Geometry: see drawing. Coordinates: mm, zero at the bounding-box minimum. Give positions to 0.01 mm unless a question says otherwise; leave off trailing zeros. Write each loop counter-clockwise with the first axis right and the second up, starting at its lowest first coordinate (ties: lowest second). Pieces come first, ordered by that corner, then holes. Notation, with made-up numbers: (66, 75) - (87, 75) arc R21 cw to (87, 113) - close; hole circle Ø9 at (7, 32). An arc over 180 degrees is marked (long way). Use a Markdown table: item, result. Add a question column.
1. Section query A-A, the plane y = 20.5. Return loops of the section in (x, z).
2. Section query B-B, the plane x = 85. Return loops of the section in (y, z).
3. Section query D-D, the plane y = 9.5. Return loops of the section in (x, z).
4. Pin query (flat end, axial travel): pin 1 (2 mm diameter, centred on x = 94.53, y = 4, fed in from -Z); pin 2 (3 mm diameter, centred on x = 85, y = 20.5, fed in from +Z). Return the tip coordinate at first contact, or that it passes through.
5. Section query C-C, the plane z = 1.05. Return loops of the section in (x, y), plus the area to 3 significant figures.
6. Material intervals for probe 1 along Y at (x, z) = (85, 0.7); probe 2 along X at (y, z) = (19.5, 0.15); probe 3 along Y at (x, z) = (94.5, 0.45), sorted ascending.
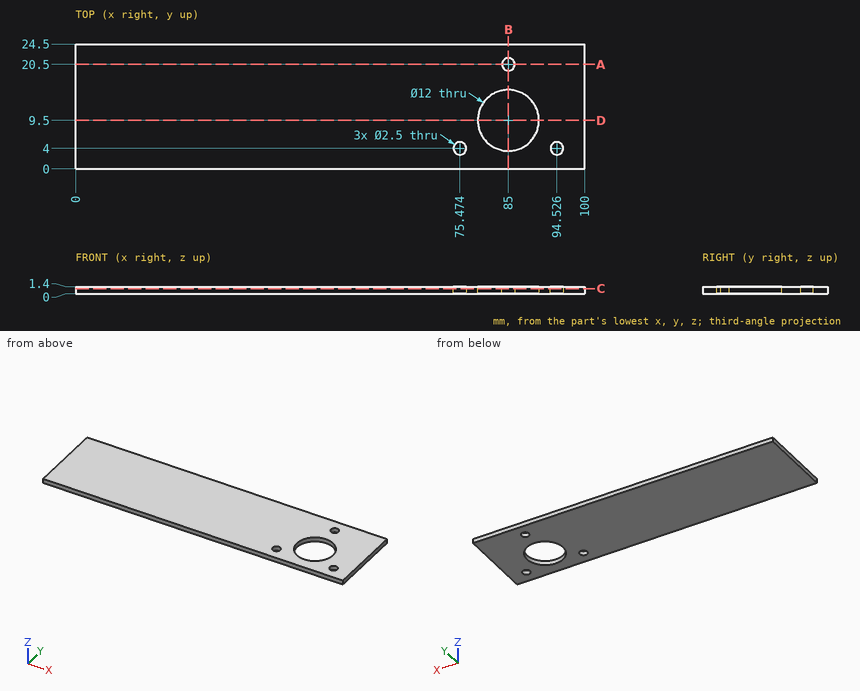
Result sheet:
| question | item | result |
|---|---|---|
| 1 | outline | (0, 0) - (83.75, 0) - (83.75, 1.4) - (0, 1.4) - close; (86.25, 0) - (100, 0) - (100, 1.4) - (86.25, 1.4) - close |
| 2 | outline | (0, 0) - (3.5, 0) - (3.5, 1.4) - (0, 1.4) - close; (15.5, 0) - (19.25, 0) - (19.25, 1.4) - (15.5, 1.4) - close; (21.75, 0) - (24.5, 0) - (24.5, 1.4) - (21.75, 1.4) - close |
| 3 | outline | (0, 0) - (79, 0) - (79, 1.4) - (0, 1.4) - close; (91, 0) - (100, 0) - (100, 1.4) - (91, 1.4) - close |
| 4 | pin 1 | passes through |
| 4 | pin 2 | stops at z = 1.4 |
| 5 | outline | (0, 0) - (100, 0) - (100, 24.5) - (0, 24.5) - close; hole circle Ø2.5 at (75.47, 4); hole circle Ø12 at (85, 9.5); hole circle Ø2.5 at (85, 20.5); hole circle Ø2.5 at (94.53, 4) |
| 5 | area | 2,320 mm² |
| 6 | probe 1 | y = 0 to 3.5, 15.5 to 19.25, 21.75 to 24.5 |
| 6 | probe 2 | x = 0 to 84.25, 85.75 to 100 |
| 6 | probe 3 | y = 0 to 2.75, 5.25 to 24.5 |
